Part model, mm, in its own coordinate system. A direction names the side the tool comes from. Round coordinates to 2 decimals unless told otherwise and drop trailing zeros. Loops run counter-clockwise (first coordinate to the right, second up) from the corner with the lowest first, then second, coordinate; pieces in that order, holes last.
1) Band-saw the part on D-D, the plane z = 13.75. Write the cut outline in (x, y), then the cut area to 3 significant figures.
2) Drop flat-ended pins along their axis: P1, Ø10, axis at x = 8, y = -14, coming from the +Z side; P2, Ø3.5, axis at x = 0, y = -9.5, coming from the +Z side; P3, Ø3.5, axis at y = -9.5, z = 6.5, coming from the +X side. Give the stop position or say it passes through.
3) Band-saw the part on C-C, the plane y = -9.5. Write the cut outline in (x, z).
4) Probe line 1 (Y direction, x = 0, z = 12.7); line 2 (Z direction, x = 10.5, y = 6.5); line 3 (X direction, y = -6, z = 6). List the from-to ranges inside material, lowest first.
5) Band-saw the part on B-B, the plane x = 0. Write the cut outline in (y, z), then the cut area to 3 significant figures.
6) Mould opens along Y. For faces 1 (the flat face through (-30, -8, 2)), 2 (the flat face through (25.762, -8, 2)), 3 (the flat face through (0, -13, 12)), 4 (the flat face through (-25.762, -7, 2)) say: +Y half, -Y half, draft (parallel to the pull), parting line (faces both ways), or undercut.
7) 3-axis set-ups, long thin cutter, end or side, ignore diameter. For faces 5 (the cylindrical face through (-10.35, -2.2, 7.55)), 6 (the cylindrical face through (23.07, 5.75, 1.97)), 7 (the flat face through (13, 1, 8)), 8 (the flat face through (-14.26, -11.986, 9.423)): which of +Z, -Z, +X, -X, +Y, -Y reach the whole face in a straight line?
from build123d import *

# Parameters (mm, degrees)
F0_W         = 30
F0_H         = 26
F1_DEPTH     = 15
F3_SIZE2     = 2
F3_SIZE      = 1.5
F5_DEPTH     = 30.001
F6_SIZE      = 4
F2_W         = 21.7
F2_H         = 7
F7_DEPTH     = 12.5
F8_W         = 11
F8_H         = 7
F9_DEPTH     = 4
F10_W        = 30
F10_H        = 5
F11_DEPTH    = 15.001
F13_D        = 4.4
F15_DEPTH    = 4
F16_SIZE     = 3.49999
F17_T4_DEPTH = 26.4149188769
F18_SIZE     = 3.49999
F19_T4_DEPTH = 26.4149188769


# Not quite as in the source:
# - a fillet or chamfer that OpenCascade refuses, or shapes differently, is made with other operations: its cross-section is extruded or revolved along the edge and cut away or added
# - a fillet or chamfer is up to 0.001 mm smaller than in the source, because OpenCascade refuses the exact size


with BuildPart() as f1:
    # F0 (on Top) → F1 (new body)
    with BuildSketch(Plane.XY):
        Rectangle(F0_W, F0_H)
    extrude(amount=F1_DEPTH)

    # F3
    f3_edges = [f1.edges().sort_by_distance(p)[0] for p in [
        (-15, -13, 7.5),
        (15, -13, 7.5),
    ]]
    f3_side = f1.faces().sort_by_distance((0, -13, 7.5))[0]
    chamfer(f3_edges, length=F3_SIZE, length2=F3_SIZE2, reference=f3_side)

    # F4 (on face) → F5 (cut, through all)
    with BuildSketch(Plane(origin=(-15, 0, 0), x_dir=(0, -1, 0), z_dir=(-1, 0, 0))):
        Polygon((-13, 12), (-13, 0), (-8, 0), (-8, 4), (-3, 4), (-3, 12), align=None)
    extrude(amount=-F5_DEPTH, mode=Mode.SUBTRACT)

    # F6
    f6_edges = [f1.edges().sort_by_distance(p)[0] for p in [
        (-15, 3, 8),
        (15, 3, 8),
    ]]
    chamfer(f6_edges, length=F6_SIZE)

    # F2 (on face) → F7 (cut)
    with BuildSketch(Plane.XZ.offset(13)):
        with Locations((0, 7.5)):
            Rectangle(F2_W, F2_H)
    extrude(amount=-F7_DEPTH, mode=Mode.SUBTRACT)

    # F8 (on face) → F9 (cut)
    with BuildSketch(Plane(origin=(0, 3, 0), x_dir=(-1, 0, 0), z_dir=(0, 1, 0))):
        with Locations((0, 7.5)):
            Rectangle(F8_W, F8_H)
    extrude(amount=-F9_DEPTH, mode=Mode.SUBTRACT)

    # F10 (on face) → F11 (cut, through all)
    with BuildSketch(Plane.XY.offset(15)):
        with Locations((0, 10.5)):
            Rectangle(F10_W, F10_H)
    extrude(amount=-F11_DEPTH, mode=Mode.SUBTRACT)

    # F13 (through all)
    with Locations(Plane.XY.offset(15)):
        with Locations((0, -9.5)):
            Hole(F13_D / 2)

    # F14 (on face) → F15 (join)
    with BuildSketch(Plane(origin=(0, 0, 0), x_dir=(1, 0, 0), z_dir=(0, 0, -1))):
        with BuildLine():
            Line((30, 23), (-30, 23))
            Line((-30, 23), (-30, 11))
            Line((-30, 11), (-25.7624481171, 11))
            Line((-25.7624481171, 11), (-25.7624481171, 18))
            ThreePointArc((-25.7624481171, 18), (-23.0124481171, 20.75), (-20.2624481171, 18))
            Line((-20.2624481171, 18), (-20.2624481171, 11))
            Line((-20.2624481171, 11), (-15, 11))
            Line((-15, 11), (-13.5, 13))
            Line((-13.5, 13), (13.5, 13))
            Line((13.5, 13), (15, 11))
            Line((15, 11), (20.2624481171, 11))
            Line((20.2624481171, 11), (20.2624481171, 18))
            ThreePointArc((20.2624481171, 18), (23.0124481171, 20.75), (25.7624481171, 18))
            Line((25.7624481171, 18), (25.7624481171, 11))
            Line((25.7624481171, 11), (30, 11))
            Line((30, 11), (30, 23))
        make_face()
        with BuildLine():
            Line((-25.7624481171, 11), (-30, 11))
            Line((-30, 11), (-30, -8))
            Line((-30, -8), (-15, -8))
            Line((-15, -8), (-15, 11))
            Line((-15, 11), (-20.2624481171, 11))
            Line((-20.2624481171, 11), (-20.2624481171, -3))
            ThreePointArc((-20.2624481171, -3), (-23.0124481171, -5.75), (-25.7624481171, -3))
            Line((-25.7624481171, -3), (-25.7624481171, 11))
        make_face()
        with BuildLine():
            Line((30, -8), (30, 11))
            Line((30, 11), (25.7624481171, 11))
            Line((25.7624481171, 11), (25.7624481171, -3))
            ThreePointArc((25.7624481171, -3), (23.0124481171, -5.75), (20.2624481171, -3))
            Line((20.2624481171, -3), (20.2624481171, 11))
            Line((20.2624481171, 11), (15, 11))
            Line((15, 11), (15, -8))
            Line((15, -8), (30, -8))
        make_face()
    extrude(amount=-F15_DEPTH)

    # F16 (size 3.5 in the source; OpenCascade refuses exactly that, so slightly less here)
    f16_edges = [f1.edges().sort_by_distance(p)[0] for p in [
        (-5.5, -0.5, 7.5),
    ]]
    chamfer(f16_edges, length=F16_SIZE)

    # F17: fillet of radius 5 on 1 edges, made by hand


with BuildPart() as f17_tool2:
    # F17_s3 → F17_t4 (new body)
    with BuildSketch(Plane.XY.offset(20.7074594385)):
        with BuildLine():
            ThreePointArc((-8.99999, -0.5), (-10.3638647521, -2.2323966462), (-10.85, -4.3829837754))
            Line((-10.85, -4.3829837754), (-10.85, -0.5))
            Line((-10.85, -0.5), (-8.99999, -0.5))
        make_face()
    extrude(amount=-F17_T4_DEPTH)

    split(bisect_by=Plane.XY.offset(15), keep=Keep.BOTTOM)

    split(bisect_by=Plane.XY, keep=Keep.TOP)


with BuildPart() as f1_1:
    add(f1.part)

    # F17_t1: union F17_tool2
    add(f17_tool2.part)

    # F18 (size 3.5 in the source; OpenCascade refuses exactly that, so slightly less here)
    f18_edges = [f1_1.edges().sort_by_distance(p)[0] for p in [
        (5.5, -0.5, 7.5),
    ]]
    chamfer(f18_edges, length=F18_SIZE)

    # F19: fillet of radius 5 on 1 edges, made by hand


with BuildPart() as f19_tool2:
    # F19_s3 → F19_t4 (new body)
    with BuildSketch(Plane.XY.offset(-5.7074594385)):
        with BuildLine():
            ThreePointArc((8.99999, -0.5), (10.3638647521, -2.2323966462), (10.85, -4.3829837754))
            Line((10.85, -4.3829837754), (10.85, -0.5))
            Line((10.85, -0.5), (8.99999, -0.5))
        make_face()
    extrude(amount=F19_T4_DEPTH)

    split(bisect_by=Plane.XY.offset(15), keep=Keep.BOTTOM)

    split(bisect_by=Plane.XY, keep=Keep.TOP)


with BuildPart() as f1_2:
    add(f1_1.part)

    # F19_t1: union F19_tool2
    add(f19_tool2.part)


solid = f1_2.part
Reported:
1. outline: (-15, -11) - (-13.5, -13) - (13.5, -13) - (15, -11) - (15, 8) - (-15, 8) - close; hole circle Ø4.4 at (0, -9.5)
1. area: 612 mm2
2. P1: stops at z = 15
2. P2: passes through
2. P3: stops at x = 15
3. outline: (-30, 0) - (-25.76, 0) - (-25.76, 4) - (-30, 4) - close; (-20.26, 0) - (-2.2, 0) - (-2.2, 4) - (-10.85, 4) - (-10.85, 11) - (-2.2, 11) - (-2.2, 15) - (-15, 15) - (-15, 4) - (-20.26, 4) - close; (2.2, 0) - (20.26, 0) - (20.26, 4) - (15, 4) - (15, 15) - (2.2, 15) - (2.2, 11) - (10.85, 11) - (10.85, 4) - (2.2, 4) - close; (25.76, 0) - (30, 0) - (30, 4) - (25.76, 4) - close
4. line 1: y = -13 to -11.7, -7.3 to 8
4. line 2: z = 0 to 4, 12 to 15
4. line 3: x = -15 to -10.85, 10.85 to 15
5. outline: (-23, 0) - (-11.7, 0) - (-11.7, 4) - (-23, 4) - close; (-13, 11) - (-11.7, 11) - (-11.7, 15) - (-13, 15) - close; (-7.3, 0) - (8, 0) - (8, 4) - (-7.3, 4) - close; (-7.3, 11) - (3, 11) - (3, 12) - (8, 12) - (8, 15) - (-7.3, 15) - close
5. area: 168 mm2
6. face 1: draft
6. face 2: undercut
6. face 3: -Y half
6. face 4: undercut
7. face 5: -Y
7. face 6: +Z, -Z
7. face 7: +X, +Y
7. face 8: +Z, -X, -Y
